Check sheet for the modelled part. Datum: model origin and axes. Units: mm. Face numbers are marked on the shaded views. A direction names the side the tool comes from. Round coordinates to 2 decimals unless told otherwise and drop trailing zeros. Order: outer loops, then holes, each group sorted by start corner. A loop starts at its lowest first (then second) coordinate and runs counter-clockwise, first axis right, second up.
(1) Depth check by flat-ended pin: pin 1 (1.1 mm diameter, centred on y = 6, z = -1.5, fed in from +X); pin 2 (2 mm diameter, centred on y = 3, z = -4, fed in from +X); pin 3 (1 mm diameter, centred on x = 2, y = 0.5, fed in from -Z). Enter the tip coordinate at first touch or a pass-through.
(2) Sectioned sample at B-B, the plane x = -11.7. Enter the section's corners in (y, z).
(3) Thickness scan on probe 1 along Y at (x, z) = (-11.7, -2.1); probe 2 along Y at (x, z) = (-6.75, -1); probe 3 along X at (y, z) = (-0.5, 0.5). Record the ranges inside material, lowest first.
(4) Sectioned sample at A-A, the plane z = -1.5. Enter the section's corners in (x, y).
(5) Tool access check on the marked faces 5, 6, 7 and 8. Record the directions out of +Z, -Z, +X, -X, +Y, -Y that give a thin tool (end or side, any length) a straight path to the whole face; none if there is none.
(6) Sectioned sample at D-D, the plane y = 2.5. Enter the section's corners in (x, z).
(7) Mould release check, pull along Y, two halves, no side actions. Record for the marked faces 1, 2, 3 and 4: released by +Y, released by -Y, zero draft, split by the parting line, or undercut.
(8) Sectioned sample at C-C, the plane y = -6. Enter the section's corners in (x, z), and give its area (3 significant figures).
```python
from build123d import *

# Parameters (mm, degrees)
BOSS_EXTRUDE1_DEPTH = 2
BOSS_EXTRUDE2_DEPTH = 5
SKETCH4_R           = 3.9
BOSS_EXTRUDE3_DEPTH = 1.2
CUT_EXTRUDE1_DEPTH  = 5
SKETCH7_W           = 1.5
SKETCH7_H           = 1.5
CUT_EXTRUDE2_DEPTH  = 5
SKETCH8_R           = 0.95
CUT_EXTRUDE3_DEPTH  = 8
SKETCH9_R           = 2
CUT_EXTRUDE4_DEPTH  = 3
SKETCH10_W          = 3
SKETCH10_H          = 1.25
CUT_EXTRUDE5_DEPTH  = 2


with BuildPart() as part:
    # Sketch1 → Boss-Extrude1 (new body)
    with BuildSketch(Plane.XY):
        with BuildLine():
            Line((-20.7, 3.793442666), (-20.7, -4.031648778))
            Line((-20.7, -4.031648778), (-15.7, -7.5))
            Line((-15.7, -7.5), (-6.7, -7.5))
            Line((-6.7, -7.5), (-4.2, -5.6))
            ThreePointArc((-4.2, -5.6), (3.130495168, -6.260990337), (7, 0))
            ThreePointArc((7, 0), (4.949747468, 4.949747468), (0, 7))
            Line((0, 7), (0, 7.5))
            Line((0, 7.5), (-16.7, 7.5))
            Line((-16.7, 7.5), (-20.7, 3.793442666))
        make_face()
    extrude(amount=BOSS_EXTRUDE1_DEPTH)

    # Sketch2 → Boss-Extrude2 (add)
    with BuildSketch(Plane(origin=(0, 0, 0), x_dir=(-1, 0, 0), z_dir=(0, 0, -1))):
        Polygon((16.7, 7.5), (20.7, 3.793442666), (20.7, -4.031648778), (15.7, -7.5), (6.7, -7.5), (6.7, -4.5), (7.7, -4.5), (7.7, 2), (5.5, 2), (5.5, 5.3), (2.5, 5.3), (2.5, 7.5), align=None)
    extrude(amount=BOSS_EXTRUDE2_DEPTH)

    # Sketch4 → Boss-Extrude3 (add)
    with BuildSketch(Plane(origin=(0, 0, 0), x_dir=(-1, 0, 0), z_dir=(0, 0, -1))):
        Circle(SKETCH4_R)
    extrude(amount=BOSS_EXTRUDE3_DEPTH)

    # Sketch5 → Cut-Extrude1 (cut)
    with BuildSketch(Plane(origin=(0, 0, -1.2), x_dir=(-1, 0, 0), z_dir=(0, 0, -1))):
        with BuildLine():
            Line((1, 0.979795897), (1, -0.979795897))
            ThreePointArc((1, -0.979795897), (-1.4, 0), (1, 0.979795897))
        make_face()
    extrude(amount=-CUT_EXTRUDE1_DEPTH, mode=Mode.SUBTRACT)

    # Sketch7 → Cut-Extrude2 (cut, along a direction that is not the sketch's normal)
    with BuildSketch(Plane.XZ.offset(7.5)):
        with Locations((-9.184228352, -5)):
            Rectangle(SKETCH7_W, SKETCH7_H)
    extrude(amount=-CUT_EXTRUDE2_DEPTH, dir=(-0.422651734, -0.906292178, 0), mode=Mode.SUBTRACT)

    # Sketch8 → Cut-Extrude3 (cut)
    with BuildSketch(Plane(origin=(0, 0, -5), x_dir=(-1, 0, 0), z_dir=(0, 0, -1))):
        with Locations((16.7, 0)):
            Circle(SKETCH8_R)
        with Locations((11.7, 0)):
            Circle(SKETCH8_R)
    extrude(amount=-CUT_EXTRUDE3_DEPTH, mode=Mode.SUBTRACT)

    # Sketch9 → Cut-Extrude4 (cut)
    with BuildSketch(Plane.XY.offset(2)):
        with Locations((-16.7, 0)):
            Circle(SKETCH9_R)
        with Locations((-11.7, 0)):
            Circle(SKETCH9_R)
    extrude(amount=-CUT_EXTRUDE4_DEPTH, mode=Mode.SUBTRACT)

    # Sketch10 → Cut-Extrude5 (cut)
    with BuildSketch(Plane(origin=(0, 0, -5), x_dir=(-1, 0, 0), z_dir=(0, 0, -1))):
        with Locations((4, 5.925)):
            Rectangle(SKETCH10_W, SKETCH10_H)
    extrude(amount=-CUT_EXTRUDE5_DEPTH, mode=Mode.SUBTRACT)


solid = part.part
```
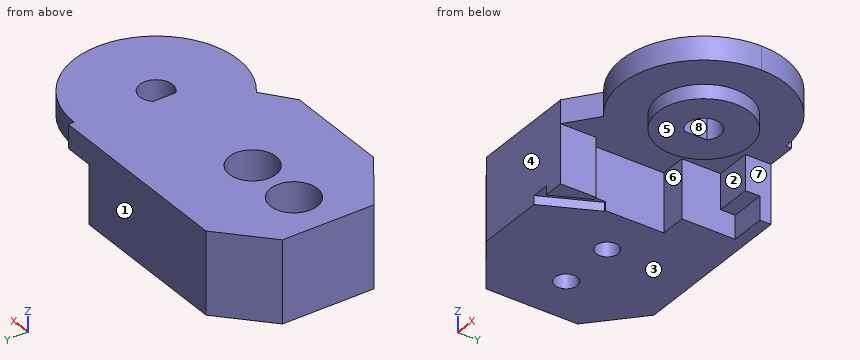
Derived:
1. pin 1: stops at x = -2.5
1. pin 2: stops at x = -5.5
1. pin 3: stops at z = -1.2
2. outline: (-7.5, -5) - (-0.95, -5) - (-0.95, -1) - (-2, -1) - (-2, 2) - (-7.5, 2) - close; (0.95, -5) - (7.5, -5) - (7.5, 2) - (2, 2) - (2, -1) - (0.95, -1) - close
3. probe 1: y = -7.5 to -0.95, 0.95 to 7.5
3. probe 2: y = -7.5 to -4.5, 2 to 7.5
3. probe 3: x = -20.7 to -18.64, -14.76 to -13.64, -9.76 to -1, 1.31 to 6.98
4. outline: (-20.7, -4.03) - (-15.7, -7.5) - (-6.7, -7.5) - (-6.7, -4.5) - (-7.7, -4.5) - (-7.7, 2) - (-5.5, 2) - (-5.5, 5.3) - (-2.5, 5.3) - (-2.5, 7.5) - (-16.7, 7.5) - (-20.7, 3.79) - close; hole circle Ø1.9 at (-16.7, 0); hole circle Ø1.9 at (-11.7, 0)
5. face 5: -Z, +X, -Y
5. face 6: -Z
5. face 7: -Z, +X, +Y
5. face 8: +Z, -Z
6. outline: (-20.7, -5) - (-5.5, -5) - (-5.5, 0) - (-2.99, 0) - (-2.99, -1.2) - (2.99, -1.2) - (2.99, 0) - (6.54, 0) - (6.54, 2) - (-20.7, 2) - close
7. face 1: released by +Y
7. face 2: undercut
7. face 3: zero draft
7. face 4: released by -Y
8. outline: (-17.86, -5) - (-9.23, -5) - (-9.23, -4.25) - (-7.73, -4.25) - (-7.73, -5) - (-6.7, -5) - (-6.7, 0) - (-4.73, 0) - (-4.73, 2) - (-17.86, 2) - close; (-3.61, 0) - (3.61, 0) - (3.61, 2) - (-3.61, 2) - close
8. area: 95.4 mm2
